Could you check a few things on this model? Use its own coordinates, in mm. Coordinates: 2 decimals unless noted, no trailing zeros. Loops run counter-clockwise (first coordinate to the right, second up) from the corner with the lowest first, then second, coordinate; pieces in that order, holes last. Notation, with made-up numbers: (41.25, 6) - (84.25, 6) arc R23 cw to (84.25, 38) - close; hole circle Ø7 at (56, -8). An arc over 180 degrees is marked (long way). One line per question, with ' | ' between items. Start each with the question number.
1. I'm going to push flat-ended pins straight in: P1, Ø2, axis at x = -7.5, y = 4, coming from the -Z side; P2, Ø11, axis at x = 65.34, z = 92.35, coming from the +Y side (3 decimals); P3, Ø3, axis at y = 4, z = -1.5, coming from the -X side; P4, Ø2, axis at x = -90, y = 3, coming from the -Z side. Where does each tip first touch, or does it pass through?
2. I want a section at A-A, the plane z = -32.5. Write out the boundary of the cut face in (x, y) (3 decimals), then the cut area to 3 significant figures.
3. I want a section at B-B, the plane x = 28. Write out the boundary of the cut face in (y, z), then the cut area to 3 significant figures.
4. Please list where these lines run through material, in increasing order: L1, parallel to X at y = 5.5, z = 43.5 (3 decimals); L2, parallel to Z at x = 12, y = 1.5; L3, parallel to Z at x = 70, y = 4. Write a range as [from, to].
5. I want a section at D-D, the plane x = -40.5. Write out the boundary of the cut face in (y, z).
6. I want a section at C-C, the plane y = 3.5. Count the separate pieces of the cut face and the enclosed holes in it, then the cut area to 3 significant figures.
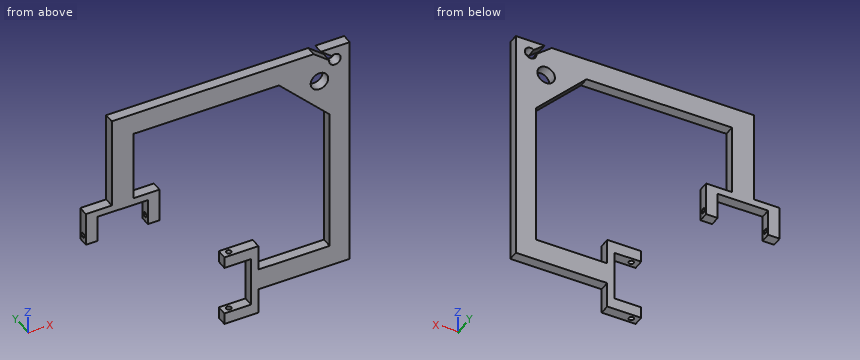
from build123d import *

# Parameters (mm, degrees)
SKETCH1_R           = 6.05
BOSS_EXTRUDE1_DEPTH = 7
SKETCH2_R           = 1.7
CUT_EXTRUDE1_DEPTH  = 60
SKETCH3_R           = 1.7
CUT_EXTRUDE2_DEPTH  = 60


with BuildPart() as part:
    # Sketch1 → Boss-Extrude1 (new body)
    with BuildSketch(Plane(origin=(0, 0, 0), x_dir=(1, 0, 0), z_dir=(0, 1, 0))):
        with BuildLine():
            Line((-87.25, -27.005178012), (-87.25, -45.345178012))
            Line((-87.25, -45.345178012), (-52.6, -45.345178012))
            Line((-52.6, -45.345178012), (-52.6, -27.005178012))
            Line((-52.6, -27.005178012), (-44.6, -27.005178012))
            Line((-44.6, -27.005178012), (-44.6, -50.345178012))
            Line((-44.6, -50.345178012), (-62.425, -50.345178012))
            Line((-62.425, -50.345178012), (-62.425, -99.345178012))
            Line((-62.425, -99.345178012), (37.575, -99.345178012))
            Line((37.575, -99.345178012), (72.34, -64.580178012))
            Line((72.34, -64.580178012), (72.34, 35.419821988))
            Line((72.34, 35.419821988), (23.34, 35.419821988))
            Line((23.34, 35.419821988), (23.34, 17.594821988))
            Line((23.34, 17.594821988), (0, 17.594821988))
            Line((0, 17.594821988), (0, 25.594821988))
            Line((0, 25.594821988), (18.34, 25.594821988))
            Line((18.34, 25.594821988), (18.34, 60.244821988))
            Line((18.34, 60.244821988), (0, 60.244821988))
            Line((0, 60.244821988), (0, 68.244821988))
            Line((0, 68.244821988), (23.34, 68.244821988))
            Line((23.34, 68.244821988), (23.34, 50.419821988))
            Line((23.34, 50.419821988), (86.165, 50.419821988))
            Line((86.165, 50.419821988), (86.165, -65.755178012))
            Line((86.165, -65.755178012), (86.165, -114.345178012))
            Line((86.165, -114.345178012), (66.299963518, -114.345178012))
            Line((66.299963518, -114.345178012), (73.771063238, -108.363510987))
            ThreePointArc((73.771063238, -108.363510987), (79.319481987, -102.911578198), (72.090531111, -105.783997211))
            Line((72.090531111, -105.783997211), (61.397619718, -114.345178012))
            Line((61.397619718, -114.345178012), (37.575, -114.345178012))
            Line((37.575, -114.345178012), (-77.425, -114.345178012))
            Line((-77.425, -114.345178012), (-77.425, -50.345178012))
            Line((-77.425, -50.345178012), (-95.25, -50.345178012))
            Line((-95.25, -50.345178012), (-95.25, -27.005178012))
            Line((-95.25, -27.005178012), (-87.25, -27.005178012))
        make_face()
        with Locations(Location((65.34, -92.345178012, 0), (0, 0, 270))):
            Circle(SKETCH1_R, mode=Mode.SUBTRACT)
    extrude(amount=BOSS_EXTRUDE1_DEPTH)

    # Sketch2 → Cut-Extrude1 (cut)
    with BuildSketch(Plane.XY.offset(-17.594821988)):
        with Locations((4.9, 3.5)):
            Circle(SKETCH2_R)
    extrude(amount=-CUT_EXTRUDE1_DEPTH, mode=Mode.SUBTRACT)

    # Sketch3 → Cut-Extrude2 (cut)
    with BuildSketch(Plane(origin=(-44.6, 0, 0), x_dir=(0, 0, -1), z_dir=(1, 0, 0))):
        with Locations((-31.905178012, 3.5)):
            Circle(SKETCH3_R)
    extrude(amount=-CUT_EXTRUDE2_DEPTH, mode=Mode.SUBTRACT)


solid = part.part
Results are:
1) P1: stops at z = 99.35 | P2: passes through | P3: stops at x = 72.34 | P4: stops at z = 27.01
2) outline: (18.34, 0) - (23.34, 0) - (23.34, 7) - (18.34, 7) - close; (72.34, 0) - (86.165, 0) - (86.165, 7) - (72.34, 7) - close | area: 132 mm2
3) outline: (0, -50.42) - (7, -50.42) - (7, -35.42) - (0, -35.42) - close; (0, 99.35) - (7, 99.35) - (7, 114.35) - (0, 114.35) - close | area: 210 mm2
4) L1: x = [-95.25, -87.25], [-52.6, -44.6], [72.34, 86.165] | L2: z = [-68.24, -60.24], [-25.59, -17.59], [99.35, 114.35] | L3: z = [-50.42, -35.42], [66.92, 88.49], [96.2, 107.46], [111.38, 114.35]
5) outline: (0, 99.35) - (7, 99.35) - (7, 114.35) - (0, 114.35) - close
6) separate pieces: 5 | enclosed holes: 1 | area: 7,380 mm2
